```python
from build123d import *

# Parameters (mm, degrees)
F0_R     = 10
F1_DEPTH = 3
F2_R     = 2
F3_R     = 7.5
F4_DEPTH = 2
F5_R     = 2.3
F6_DEPTH = 6.5


with BuildPart() as f1:
    # F0 (on Top) → F1 (new body)
    with BuildSketch(Plane.XY):
        Circle(F0_R)
    extrude(amount=F1_DEPTH)

    # F2
    f2_edges = [f1.edges().sort_by_distance(p)[0] for p in [
        (-10, 0, 0),
    ]]
    fillet(f2_edges, radius=F2_R)

    # F3 (on face) → F4 (join)
    with BuildSketch(Plane.XY.offset(3)):
        Circle(F3_R)
    extrude(amount=F4_DEPTH)

    # F5 (on face) → F6 (join)
    with BuildSketch(Plane.XY.offset(5)):
        Circle(F5_R)
    extrude(amount=F6_DEPTH)


solid = f1.part
```
Geometry check sheet. Reference: the model listing, model coordinates, mm. A direction names the side the tool comes from. Coordinates: 2 decimals unless noted, no trailing zeros. Loops run counter-clockwise (first coordinate to the right, second up) from the corner with the lowest first, then second, coordinate; pieces in that order, holes last. Notation, with made-up numbers: (47, 22) -> (93, 22) arc R23 cw to (93, 44) -> close; hole circle Ø6 at (51, 3.5). An arc over 180 degrees is marked (long way). Put each result on its own line as item: value.
1) Cross-section at C-C on z = 2.5. Record the boundary of the cut face in (x, y), plus the area to 3 significant figures.
Result set:
outline: circle Ø20 at (0, 0)
area: 314 mm^2
2) Gauge pin test, flat ends, axial feed: pin 1 Ø6 at (x, z) = (5, 9.5) entering from -Y; pin 2 Ø2 at (x, y) = (7, -5.5) entering from +Z; pin 3 Ø6 at (x, y) = (-3, -7) entering from +Z. Record the tip position at first contact, or that the pin passes through.
Result set:
pin 1: stops at y = -1.14
pin 2: stops at z = 3
pin 3: stops at z = 5
3) Cross-section at D-D on z = 5.25. Record the boundary of the cut face in (x, y), plus the area to 3 significant figures.
Result set:
outline: circle Ø4.6 at (0, 0)
area: 16.6 mm^2
4) Tool access check on faces 1 (the flat face through (0, 0, 11.5)), 2 (the flat face through (4, 7, 3)). Record the directions out of +Z, -Z, +X, -X, +Y, -Y that give a thin tool (end or side, any length) a straight path to the whole face; none if there is none.
Result set:
face 1: +Z, +X, -X, +Y, -Y
face 2: +Z
5) Cross-section at A-A on x = 0. Record the boundary of the cut face in (y, z).
Result set:
outline: (-10, 2) arc R2 ccw to (-8, 0) -> (8, 0) arc R2 ccw to (10, 2) -> (10, 3) -> (7.5, 3) -> (7.5, 5) -> (2.3, 5) -> (2.3, 11.5) -> (-2.3, 11.5) -> (-2.3, 5) -> (-7.5, 5) -> (-7.5, 3) -> (-10, 3) -> close
6) Thickness scan on line 1 (Z direction, x = -1.5, y = -7.75); line 2 (Z direction, x = 2.75, y = 1); line 3 (X direction, y = 7, z = 1.5). Record the ranges inside material, lowest first.
Result set:
line 1: z = 0 to 3
line 2: z = 0 to 5
line 3: x = -7.05 to 7.05
